```python
from build123d import *

# Parameters (mm, degrees)
F0_W     = 97.735152
F0_H     = 88.60518
F0_R     = 36.927875
F1_DEPTH = 24.485806
F2_R     = 5.08
F3_R     = 7.709535
F4_DEPTH = 25.4
F5_R     = 2.54


with BuildPart() as f1:
    # F0 (on Front) → F1 (new body)
    with BuildSketch(Plane.XZ):
        Rectangle(F0_W, F0_H)
        Circle(F0_R, mode=Mode.SUBTRACT)
    extrude(amount=F1_DEPTH)

    # F2
    f2_edges = [f1.edges().sort_by_distance(p)[0] for p in [
        (48.867576, -12.242903, 44.30259),
        (48.867576, -12.242903, -44.30259),
        (-48.867576, -12.242903, 44.30259),
        (-48.867576, -12.242903, -44.30259),
    ]]
    fillet(f2_edges, radius=F2_R)

    # F3 (on face) → F4 (cut)
    with BuildSketch(Plane.YZ.offset(48.867576)):
        with Locations((-11.589006, 0)):
            Circle(F3_R)
    extrude(amount=-F4_DEPTH, mode=Mode.SUBTRACT)

    # F5
    f5_edges = [f1.edges().sort_by_distance(p)[0] for p in [
        (-36.927875, -24.485806, 0),
    ]]
    fillet(f5_edges, radius=F5_R)


solid = f1.part
```
Model file for the job. Use its own axes, mm. Round coordinates to 2 decimals unless told otherwise and drop trailing zeros. Loops run counter-clockwise (first coordinate to the right, second up) from the corner with the lowest first, then second, coordinate; pieces in that order, holes last. Notation, with made-up numbers: M 15,53 L 57,53 A17 ccw 57,63 Z; hole C 69.25,82.5 d11. An arc over 180 degrees is marked long. Put each result on its own line as item: value. Start each with the question number.
Item 1: Cut at A-A (x = 0). List the corners of the cut face in (y, z).
Item 2: Drop a flat-ended pin along its axis: P1, Ø4, axis at x = 37.5, z = 4, coming from the +Y side. Give the stop position or say it passes through.
Item 3: Cut at B-B (z = 0). List the corners of the cut face in (x, y).
Item 4: Cut at C-C (y = -16). List the corners of the cut face in (x, z).
Item 5: Drill centre lines: line 1 along Z through (x, y) = (0, -4.75); line 2 along Z through (x, y) = (27, -23.5); line 3 along X through (y, z) = (-20, -5.5). Where is each one in solid material? Low to high.
Item 6: Mould opens along Z. For faces 1 (the face through (-1, -12, -44.303)), 2 (the face through (-1, -24.486, 40)), 3 (the face through (42.58, -4.467, -2.953)) say: released by +Z, released by -Z, zero draft, split by the parting line, or undercut.
Item 7: Cut at D-D (y = -9.5). List the corners of the cut face in (x, z), then the cut area to 3 significant figures.
Answer block:
1. outline: M -24.49,-44.3 L 0,-44.3 L 0,-36.93 L -21.95,-36.93 A2.54 ccw -24.49,-39.47 Z; M -24.49,39.47 A2.54 ccw -21.95,36.93 L 0,36.93 L 0,44.3 L -24.49,44.3 Z
2. P1: y = 0
3. outline: M -48.87,-24.49 L -39.47,-24.49 A2.54 ccw -36.93,-21.95 L -36.93,0 L -48.87,0 Z; M 36.93,-21.95 A2.54 ccw 39.47,-24.49 L 48.87,-24.49 L 48.87,-19.3 L 36.93,-19.3 Z; M 36.93,-3.88 L 48.87,-3.88 L 48.87,0 L 36.93,0 Z
4. outline: M -48.87,-39.22 A5.08 ccw -43.79,-44.3 L 43.79,-44.3 A5.08 ccw 48.87,-39.22 L 48.87,-6.32 L 36.38,-6.32 A36.93 cw long 36.38,6.32 L 48.87,6.32 L 48.87,39.22 A5.08 ccw 43.79,44.3 L -43.79,44.3 A5.08 ccw -48.87,39.22 Z
5. line 1: -44.3 to -36.93, 36.93 to 44.3
5. line 2: -44.3 to -25.96, 25.96 to 44.3
5. line 3: -48.87 to -36.52, 36.52 to 48.87
6. face 1: released by -Z
6. face 2: zero draft
6. face 3: undercut
7. outline: M -48.87,-39.22 A5.08 ccw -43.79,-44.3 L 43.79,-44.3 A5.08 ccw 48.87,-39.22 L 48.87,-7.42 L 36.17,-7.42 A36.93 cw long 36.17,7.42 L 48.87,7.42 L 48.87,39.22 A5.08 ccw 43.79,44.3 L -43.79,44.3 A5.08 ccw -48.87,39.22 Z
7. area: 4,170 mm2
